from build123d import *

# Parameters (mm, degrees)
SKETCH_1_W          = 70
SKETCH_1_H          = 70
SKETCH_1_R          = 1.7
EXTRUDE_1_DEPTH     = 2
FILLET_1_R          = 2
SKETCH_2_R          = 2.5
SKETCH_2_R_2        = 1.7
CUT_EXTRUDE_1_DEPTH = 0.5


with BuildPart() as part:
    # 草图1 → 凸台-拉伸1 (new body)
    with BuildSketch(Plane(origin=(0, 0, 0), x_dir=(1, 0, 0), z_dir=(0, 1, 0))):
        with Locations((-3.5, 3.5)):
            Rectangle(SKETCH_1_W, SKETCH_1_H)
        with Locations(Location((-28, -28, 0), (0, 0, 270))):
            Circle(SKETCH_1_R, mode=Mode.SUBTRACT)
        with Locations(Location((28, -28, 0), (0, 0, 270))):
            Circle(SKETCH_1_R, mode=Mode.SUBTRACT)
        with Locations(Location((28, 28, 0), (0, 0, 270))):
            Circle(SKETCH_1_R, mode=Mode.SUBTRACT)
        with Locations(Location((-28, 28, 0), (0, 0, 270))):
            Circle(SKETCH_1_R, mode=Mode.SUBTRACT)
        with Locations(Location((28, 35, 0), (0, 0, 270))):
            Circle(SKETCH_1_R, mode=Mode.SUBTRACT)
        with Locations(Location((-35, -28, 0), (0, 0, 90))):
            Circle(SKETCH_1_R, mode=Mode.SUBTRACT)
        with Locations(Location((-35, 35, 0), (0, 0, 90))):
            Circle(SKETCH_1_R, mode=Mode.SUBTRACT)
    extrude(amount=EXTRUDE_1_DEPTH)

    # 圆角1
    fillet_1_edges = [part.edges().sort_by_distance(p)[0] for p in [
        (-38.5, 1, -38.5),
        (31.5, 1, -38.5),
        (31.5, 1, 31.5),
        (-38.5, 1, 31.5),
    ]]
    fillet(fillet_1_edges, radius=FILLET_1_R)

    # 草图2 → 切除-拉伸1 (cut)
    # profile 1 of 7: a face of its own
    with BuildSketch(Plane.XZ):
        with Locations(Location((-28, 28, 0), (0, 0, 270))):
            Circle(SKETCH_2_R)
        with Locations(Location((-28, 28, 0), (0, 0, 270))):
            Circle(SKETCH_2_R_2, mode=Mode.SUBTRACT)
    # profile 2 of 7: a face of its own
    with BuildSketch(Plane.XZ):
        with Locations(Location((-35, 28, 0), (0, 0, 270))):
            Circle(SKETCH_2_R)
        with Locations(Location((-35, 28, 0), (0, 0, 270))):
            Circle(SKETCH_2_R_2, mode=Mode.SUBTRACT)
    # profile 3 of 7: a face of its own
    with BuildSketch(Plane.XZ):
        with Locations(Location((28, 28, 0), (0, 0, 270))):
            Circle(SKETCH_2_R)
        with Locations(Location((28, 28, 0), (0, 0, 270))):
            Circle(SKETCH_2_R_2, mode=Mode.SUBTRACT)
    # profile 4 of 7: a face of its own
    with BuildSketch(Plane.XZ):
        with Locations(Location((28, -28, 0), (0, 0, 270))):
            Circle(SKETCH_2_R)
        with Locations(Location((28, -28, 0), (0, 0, 270))):
            Circle(SKETCH_2_R_2, mode=Mode.SUBTRACT)
    # profile 5 of 7: a face of its own
    with BuildSketch(Plane.XZ):
        with Locations(Location((28, -35, 0), (0, 0, 270))):
            Circle(SKETCH_2_R)
        with Locations(Location((28, -35, 0), (0, 0, 270))):
            Circle(SKETCH_2_R_2, mode=Mode.SUBTRACT)
    # profile 6 of 7: a face of its own
    with BuildSketch(Plane.XZ):
        with Locations(Location((-28, -28, 0), (0, 0, 270))):
            Circle(SKETCH_2_R)
        with Locations(Location((-28, -28, 0), (0, 0, 270))):
            Circle(SKETCH_2_R_2, mode=Mode.SUBTRACT)
    # profile 7 of 7: a face of its own
    with BuildSketch(Plane.XZ):
        with Locations(Location((-35, -35, 0), (0, 0, 270))):
            Circle(SKETCH_2_R)
        with Locations(Location((-35, -35, 0), (0, 0, 270))):
            Circle(SKETCH_2_R_2, mode=Mode.SUBTRACT)
    extrude(amount=-CUT_EXTRUDE_1_DEPTH, mode=Mode.SUBTRACT)


solid = part.part
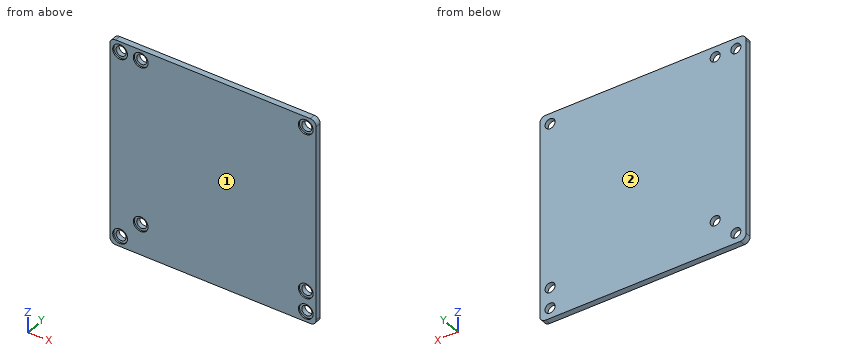
Here's how the part is built. I have some questions about the finished solid (model axes, mm). Face numbers are marked on the shaded views. Coordinates: 2 decimals unless noted, no trailing zeros. Write each loop counter-clockwise with the first axis right and the second up, starting at its lowest first coordinate (ties: lowest second). Pieces come first, ordered by that corner, then holes.
Item 1: If we mould it in two halves opening along Y, with no side actions, what happens to the marked faces 1 and 2? For each: +Y half, -Y half, draft (parallel to the pull), parting line (faces both ways), or undercut.
Item 2: I want a section at B-B on z = 28. Write out the boundary of the cut face in (x, y).
Item 3: Will this pin go through, and if not, where does the flat tip stop? pin 1 (4.5 mm diameter, centred on x = -28, z = -28, fed in from -Y).
Item 4: I want a section at A-A on x = 28. Write out the boundary of the cut face in (y, z), and give its area (3 significant figures).
Item 5: I want a section at D-D on x = -35. Write out the boundary of the cut face in (y, z), and give its area (3 significant figures).
Item 6: If I drill on line 1 (X direction, y = 1, z = -28); line 2 (X direction, y = 1.65, z = 28); line 3 (Z direction, x = -35, y = 1.35), over which ranges is the centre line in solid material (lowest first)?
Item 7: I want a section at C-C on z = -28. Write out the boundary of the cut face in (x, y), and give its area (3 significant figures).
Findings below:
1. face 1: -Y half
1. face 2: +Y half
2. outline: (-38.5, 0) - (-37.5, 0) - (-37.5, 0.5) - (-36.7, 0.5) - (-36.7, 2) - (-38.5, 2) - close; (-33.3, 0.5) - (-32.5, 0.5) - (-32.5, 0) - (-30.5, 0) - (-30.5, 0.5) - (-29.7, 0.5) - (-29.7, 2) - (-33.3, 2) - close; (-26.3, 0.5) - (-25.5, 0.5) - (-25.5, 0) - (25.5, 0) - (25.5, 0.5) - (26.3, 0.5) - (26.3, 2) - (-26.3, 2) - close; (29.7, 0.5) - (30.5, 0.5) - (30.5, 0) - (31.5, 0) - (31.5, 2) - (29.7, 2) - close
3. pin 1: stops at y = 0.5
4. outline: (0, -38.5) - (2, -38.5) - (2, -36.7) - (0.5, -36.7) - (0.5, -37.5) - (0, -37.5) - close; (0, -32.5) - (0.5, -32.5) - (0.5, -33.3) - (2, -33.3) - (2, -29.7) - (0.5, -29.7) - (0.5, -30.5) - (0, -30.5) - close; (0, -25.5) - (0.5, -25.5) - (0.5, -26.3) - (2, -26.3) - (2, 26.3) - (0.5, 26.3) - (0.5, 25.5) - (0, 25.5) - close; (0, 30.5) - (0.5, 30.5) - (0.5, 29.7) - (2, 29.7) - (2, 31.5) - (0, 31.5) - close
4. area: 117 mm2
5. outline: (0, -38.5) - (2, -38.5) - (2, -36.7) - (0.5, -36.7) - (0.5, -37.5) - (0, -37.5) - close; (0, -32.5) - (0.5, -32.5) - (0.5, -33.3) - (2, -33.3) - (2, 26.3) - (0.5, 26.3) - (0.5, 25.5) - (0, 25.5) - close; (0, 30.5) - (0.5, 30.5) - (0.5, 29.7) - (2, 29.7) - (2, 31.5) - (0, 31.5) - close
5. area: 125 mm2
6. line 1: x = -38.5 to -29.7, -26.3 to 26.3, 29.7 to 31.5
6. line 2: x = -38.5 to -36.7, -33.3 to -29.7, -26.3 to 26.3, 29.7 to 31.5
6. line 3: z = -38.5 to -36.7, -33.3 to 26.3, 29.7 to 31.5
7. outline: (-38.5, 0) - (-30.5, 0) - (-30.5, 0.5) - (-29.7, 0.5) - (-29.7, 2) - (-38.5, 2) - close; (-26.3, 0.5) - (-25.5, 0.5) - (-25.5, 0) - (25.5, 0) - (25.5, 0.5) - (26.3, 0.5) - (26.3, 2) - (-26.3, 2) - close; (29.7, 0.5) - (30.5, 0.5) - (30.5, 0) - (31.5, 0) - (31.5, 2) - (29.7, 2) - close
7. area: 125 mm2
